```python
from build123d import *

# Parameters (mm, degrees)
DODANIE_WYCI_GNI_CIE1_DEPTH = 40
ZAOKR_GLENIE1_R             = 20
SZKIC6_R                    = 3
WYTNIJ_WYCI_GNI_CIE1_DEPTH  = 10
WYTNIJ_WYCI_GNI_CIE2_DEPTH  = 69.190908485


with BuildPart() as part:
    # Szkic1 → Dodanie-wyciągnięcie1 (new body)
    with BuildSketch(Plane.XY):
        Polygon((0, 0), (-5, 0), (-5, 55), (0, 55), (0, 51.5), align=None)
    extrude(amount=DODANIE_WYCI_GNI_CIE1_DEPTH)

    # Zaokrąglenie1
    zaokr_glenie1_edges = [part.edges().sort_by_distance(p)[0] for p in [
        (-2.5, 0, 0),
        (-2.5, 0, 40),
    ]]
    fillet(zaokr_glenie1_edges, radius=ZAOKR_GLENIE1_R - 0.0001)  # a hair under: the kernel refuses the full size

    # Szkic6 → Wytnij-wyciągnięcie1 (cut)
    with BuildSketch(Plane.ZY.offset(5)):
        with Locations((20, 21.237598079)):
            Circle(SZKIC6_R)
    extrude(amount=-WYTNIJ_WYCI_GNI_CIE1_DEPTH, mode=Mode.SUBTRACT)

    # Szkic8 → Wytnij-wyciągnięcie2 (cut, through all)
    with BuildSketch(Plane.ZY.offset(5)):
        Polygon((0, 50), (9, 50), (9, 55), (17.366037593, 55), (17.366037593, 50), (25.366037593, 50), (25.366037593, 55), (33, 55), (33, 50), (40, 50), (40, 57.074314744), (0, 57.074314744), align=None)
    extrude(amount=-WYTNIJ_WYCI_GNI_CIE2_DEPTH, mode=Mode.SUBTRACT)


solid = part.part
```
Design review of the part built by this model. Coordinates are the model's own, in mm. A direction names the side the tool comes from. Round coordinates to 2 decimals unless told otherwise and drop trailing zeros. Write each loop counter-clockwise with the first axis right and the second up, starting at its lowest first coordinate (ties: lowest second). Pieces come first, ordered by that corner, then holes.
Item 1: The part is to be moulded in two halves that separate along Z. For faces 4 (the flat face through (0, 27, 20)), 5 (the flat face through (-2, 35, 0)), 6 (the flat face through (-3, 53, 17.366)), 7 (the flat face through (-3, 50, 21)), say which applies: +Z half, -Z half, draft (parallel to the pull), parting line (faces both ways), or undercut.
Item 2: We need section B-B on z = 3.5. Write out the cut boundary in (x, y).
Item 3: We need section C-C on z = 30. Write out the cut boundary in (x, y), and give its area (3 significant figures).
Item 4: For faces 1 (the flat face through (-3, 50, 36)), 2 (the flat face through (-3, 52, 9)), 3 (the flat face through (-3, 52, 25.366)), list the 3-axis set-ups (+Z, -Z, +X, -X, +Y, -Y) from which the entire face can be reached by the end or side of a thin tool; tool diameter is ignored.
Item 5: For probe 1 along Y at (x, z) = (-3.9, 20); probe 2 along Z at (x, y) = (-3.95, 51); probe 3 along Y at (x, z) = (-3.45, 18.5), list the stretches that pass through material, from the lowest coordinate up.
Item 6: Clearance check with flat-ended pins moving along their axes: pin 1 Ø1.5 at (x, y) = (-2, 51.5) entering from +Z; pin 2 Ø2.5 at (x, z) = (-1.5, 23) entering from +Y; pin 3 Ø1.5 at (x, y) = (-1.5, 53.5) entering from -Z. State where each tip first meets the part, or that it passes through.
Returned:
1. face 4: draft
1. face 5: -Z half
1. face 6: undercut
1. face 7: undercut
2. outline: (-5, 8.7) - (0, 8.7) - (0, 50) - (-5, 50) - close
3. outline: (-5, 2.68) - (0, 2.68) - (0, 55) - (-5, 55) - close
3. area: 262 mm2
4. face 1: +Z, +X, -X, +Y
4. face 2: -Z, +X, -X, +Y
4. face 3: +X, -X, +Y
5. probe 1: y = 0 to 18.24, 24.24 to 50
5. probe 2: z = 9 to 17.37, 25.37 to 33
5. probe 3: y = 0.06 to 18.64, 23.84 to 50
6. pin 1: stops at z = 33
6. pin 2: stops at y = 50
6. pin 3: stops at z = 9
